Autodesk Inventor part; units mm, degrees
ref_plane "YZ Plane" through (0, 0, 0) normal (1, 0, 0) x (0, 1, 0)
ref_plane "XZ Plane" through (0, 0, 0) normal (0, 1, 0) x (-1, 0, 0)
ref_plane "XY Plane" through (0, 0, 0) normal (0, 0, 1) x (1, 0, 0)
sketch "Náčrt1" plane through (0, 0, 0) normal (0, 1, 0) x (-1, 0, 0)
  line L0 (0, 0) -> (0, -15)
  line L1 (10, 0) -> (10, -15)
  line L2 (6, -5) -> (4, -5)
  line L3 (10, -15) -> (0, -15)
  line L4 (6, -5) -> (8, 0)
  line L5 (8, 0) -> (10, 0)
  line L6 (4, -5) -> (2, 0)
  line L7 (2, 0) -> (0, 0)
  dimension "d0" = 2
  dimension "d1" = 5
  dimension "d2" = 15
  dimension "d5" = 2
  dimension "d6" = 10
revolve "Rotace1" add sketch "Náčrt1" angle 360 about axis through (-10, 0, -15) along (1, 0, 0)
sketch "Náčrt2" plane through (0, 0, -15) normal (1, 0, 0) x (0, 0, -1)
  circle A0 centre (0, 0) radius 15
  circle A1 centre (0, 0) radius 10
  circle A2 centre (0, 0) radius 10.5
  point P0 (-15, 0)
  dimension "d8" = 21
extrude "Vysunutí1" cut sketch "Náčrt2" against normal blind 2.3 contours A1 | A2
sketch "Náčrt3" plane through (-10, 0, -15) normal (-1, 0, 0) x (0, 0, 1)
  circle A0 centre (0, 0) radius 15
  circle A1 centre (0, 0) radius 3
  point P0 (15, 0)
  dimension "d11" = 6
extrude "Vysunutí2" cut sketch "Náčrt3" against normal blind 3 contours A1
sketch "Náčrt4" plane through (-7, 0, -15) normal (-1, 0, 0) x (0, 0, 1)
  circle A0 centre (0, 0) radius 15
  circle A1 centre (0, 0) radius 10
  circle A2 centre (0, 0) radius 1.5
  point P0 (15, 0)
  dimension "d14" = 3
extrude "Vysunutí3" cut sketch "Náčrt4" against normal through all contours A2
sketch "Náčrt5" plane through (-10, 0, -15) normal (-1, 0, 0) x (0, 0, 1)
  circle A0 centre (0, 0) radius 3
  circle A1 centre (0, 0) radius 15
  circle A2 centre (0, 0) radius 1.5 construction
  circle A3 centre (0, 0) radius 7 construction
  circle A4 centre (7, 0) radius 1.4
  circle A5 centre (0, 0) radius 10 construction
  circle A6 centre (10, 0) radius 0.5
  circle A7 centre (0, 0) radius 15 construction
  line L0 (0, 15) -> (0, -15) construction
  circle A8 centre (-7, 0) radius 1.4
  point P0 (15, 0)
  dimension "d17" = 8
  dimension "d18" = 2.8
  dimension "d21" = 5
  dimension "d22" = 1
extrude "Vysunutí4" cut sketch "Náčrt5" against normal through all contours A4 | A6 | A8
sketch "Náčrt6" plane through (-10, 0, -15) normal (-1, 0, 0) x (0, 0, 1)
  circle A0 centre (7, 0) radius 1.4
  circle A1 centre (10, 0) radius 0.5
  circle A2 centre (0, 0) radius 3
  circle A3 centre (0, 0) radius 15
  point P0 (15, 0)
ref_plane "Pracovní rovina1" through (-6, 0, -15) normal (-1, 0, 0) x (0, 0, 1)
split "Rozdělit1" plane through (-6, 0, -15) removes the side toward (-1, 0, 0)
sketch "Sketch7" plane through (-6, 0, -15) normal (-1, 0, 0) x (0, 0, 1)
  circle A0 centre (-7, 0) radius 1.5
  circle A1 centre (7, 0) radius 1.4
  arc A2 (9.9875, 0.4998) -> (9.9875, -0.4998) centre (10, 0) ccw
  arc A3 (9.9875, 0.4998) -> (9.9875, -0.4998) centre (0, 0) ccw
  circle A4 centre (0, 0) radius 1.5
  point P0 (15, 0)
extrude "Extrusion5" cut sketch "Sketch7" against normal blind 1 contours A0 | A1 | A2 A3 | A4
properties part number "bubinek_BOTTOM"
Can you work these out from the model? Positions are in its coordinate system, mm. A direction names the side the tool comes from. Give positions to 0.01 mm unless a question says otherwise; leave off trailing zeros. Order: outer loops, then holes, each group sorted by start corner. A loop starts at its lowest first (then second) coordinate and runs counter-clockwise, first axis right, second up. Notation, with made-up numbers: M 36,21 L 42,21 A17 cw 42,41 Z; hole C 16.25,10 d10. An arc over 180 degrees is marked long. Use a Markdown table: item, result. Add a question column.
Item 1: We'd pull the mould along Z, two halves only. Please class faces 4 (the flat face through (-5, 0, -13)), 5 (the conical face through (-3.875, -0.453, -25.303)), 6 (the cylindrical face through (-3.4, 0, -5.5)): +Z half, -Z half, draft (parallel to the pull), parting line (faces both ways), or undercut.
Item 2: For faces 1 (the cylindrical face through (-1.1, 3.2, -25)), 2 (the cylindrical face through (-3.67, 0.07, -16.5)), 3 (the cylindrical face through (-4.49, -0.43, -24.99)), which set-ups out of +Z, -Z, +X, -X, +Y, -Y let a thin tool reach every point of the face, with its end or its side?
Item 3: Will these pins go through, and if not, where does the flat tip stop? pin 1 (10.5 mm diameter, centred on y = 3, z = -18, fed in from +X); pin 2 (6 mm diameter, centred on y = -12, z = -26.5, fed in from -X); pin 3 (1.5 mm diameter, centred on x = -1.5, y = -1.5, fed in from -Z); pin 4 (1.7 mm diameter, centred on y = 0, z = -22, fed in from +X).
Item 4: Suppose I cut it at C-C (x = -1.05). List the corners of the cut face in (y, z) for me, then the cut area to 3 significant figures.
Item 5: If I drill on L1, parallel to Y at x = -0.65, z = -15; L2, parallel to Y at x = -4.35, z = -15; L3, parallel to X at y = 2, z = -14, over which ranges is the centre line in solid material (lowest first)? Write a range as [from, to].
Item 6: Suppose I cut it at A-A (z = -15). List the corners of the cut face in (x, y) for me, then the cut area to 3 significant figures.
Item 7: Suppose I cut it at B-B (x = -2.75). List the corners of the cut face in (y, z) for me (3 decimals).
Answer sheet:
| question | item | result |
|---|---|---|
| 1 | face 4 | draft |
| 1 | face 5 | parting line |
| 1 | face 6 | undercut |
| 2 | face 1 | +X |
| 2 | face 2 | +X, -X |
| 2 | face 3 | -X |
| 3 | pin 1 | stops at x = -2.3 |
| 3 | pin 2 | stops at x = -2.55 |
| 3 | pin 3 | stops at z = -29.98 |
| 3 | pin 4 | passes through |
| 4 | outline | C 0,-15 d30; hole C 0,-15 d21 |
| 4 | area | 360 mm² |
| 5 | L1 | y = [-15, -10.5], [10.5, 15] |
| 5 | L2 | y = [-10, -1.5], [1.5, 10] |
| 5 | L3 | x = [-5, -2.3] |
| 6 | outline | M -5,-10 L -4,-10 L -2,-15 L 0,-15 L 0,-10.5 L -2.3,-10.5 L -2.3,-1.5 L -5,-1.5 Z; M -5,1.5 L -2.3,1.5 L -2.3,10.5 L 0,10.5 L 0,15 L -2,15 L -4,10 L -5,10 Z |
| 6 | area | 73.6 mm² |
| 7 | outline | C 0,-15 d26.25; hole C 0,-15 d3; hole C 0,-22 d2.8; hole C 0,-8 d2.8; hole C 0,-5 d1 |
